Part model, mm, in its own coordinate system. A direction names the side the tool comes from. Coordinates: 2 decimals unless noted, no trailing zeros. Loops run counter-clockwise (first coordinate to the right, second up) from the corner with the lowest first, then second, coordinate; pieces in that order, holes last. Notation, with made-up numbers: M 78,81 L 110,81 A28 ccw 110,108 Z; hole C 28,29 d2. An arc over 180 degrees is marked long. Answer as a JSON object with one key per item and string values. Group by question number.
1. 3-axis set-ups, long thin cutter, end or side, ignore diameter. For faces 1 (the face through (-22.024, -6.007, -19.076)), 2 (the face through (-23, 5, 0)), 3 (the face through (39.634, 5.362, -12.932)), 4 (the face through (60.171, 0, 0)), 5 (the face through (14.57, 19.961, -10.382)): which of +Z, -Z, +X, -X, +Y, -Y reach the whole face in a straight line?
2. Drop flat-ended pins along their axis: pin 1 Ø8 at (x, y) = (33, -13.5) entering from -Z; pin 2 Ø8 at (x, z) = (-34, -16) entering from -Y; pin 3 Ø8 at (x, y) = (6, 15.5) entering from +Z. Give the stop position or say it passes through.
3. Saw through at C-C on x = -36.5. Write the cut outline in (y, z), then the cut area to 3 significant figures.
4. Saw through at B-B on z = 0. Write the cut outline in (x, y).
5. Drill centre lines: L1, parallel to X at y = 2.5, z = -3; L2, parallel to X at y = 3.5, z = 15; L3, parallel to Y at x = -2.5, z = -10. Where is each one in solid material? Low to high.
6. Saw through at D-D on z = 7.5. Write the cut outline in (x, y).
7. Saw through at A-A on y = 0. Write the cut outline in (x, z), then the cut area to 3 significant figures.
from build123d import *

# Parameters (mm, degrees)
CUT_EXTRUDE1_DEPTH      = 69.066884873
CUT_EXTRUDE1_DEPTH_BACK = 69.066884873
SKETCH2_W               = 43
SKETCH2_H               = 10


with BuildPart() as part:
    # Sketch1 → Revolve1 (revolve)
    with BuildSketch(Plane(origin=(0, 0, 0), x_dir=(1, 0, 0), z_dir=(0, 1, 0))):
        Polygon((-55.485714286, 0), (-55.485714286, 20), (10.514285714, 20), (10.514285714, 22.5), (18.514285714, 22.5), (18.514285714, 14), (60.171428571, 14), (60.171428571, 0), align=None)
    revolve(axis=Axis((60.171428571, 0, 0), (-1, 0, 0)))

    # Sketch2 → Cut-Extrude1 (cut, two sides: drawn at the far end of the back side and taken through both)
    with BuildSketch(Plane.XY.offset(-CUT_EXTRUDE1_DEPTH_BACK)):
        with Locations((-22.985714286, 0)):
            Rectangle(SKETCH2_W, SKETCH2_H)
    extrude(amount=CUT_EXTRUDE1_DEPTH + CUT_EXTRUDE1_DEPTH_BACK, mode=Mode.SUBTRACT)


solid = part.part
Outcome:
{
 "1": {"face 1": "-X", "face 2": "+Z, -Z", "face 3": "+X", "face 4": "+Z, -Z, +X, +Y, -Y", "face 5": "+X, -X"},
 "2": {"pin 1": "stops at z = -10.28", "pin 2": "stops at y = -16", "pin 3": "stops at z = 16.36"},
 "3": {"outline": "M -5,-19.36 L -5,19.36 A20 ccw Z; M 5,-19.36 A20 ccw 5,19.36 Z", "area": "861 mm²"},
 "4": {"outline": "M -55.49,-20 L 10.51,-20 L 10.51,-22.5 L 18.51,-22.5 L 18.51,-14 L 60.17,-14 L 60.17,14 L 18.51,14 L 18.51,22.5 L 10.51,22.5 L 10.51,20 L -55.49,20 Z; hole M -44.49,-5 L -1.49,-5 L -1.49,5 L -44.49,5 Z"},
 "5": {"L1": "x = -55.49 to -44.49, -1.49 to 60.17", "L2": "x = -55.49 to -44.49, -1.49 to 18.51", "L3": "y = -17.32 to -5, 5 to 17.32"},
 "6": {"outline": "M -55.49,-18.54 L 10.51,-18.54 L 10.51,-21.21 L 18.51,-21.21 L 18.51,-11.82 L 60.17,-11.82 L 60.17,11.82 L 18.51,11.82 L 18.51,21.21 L 10.51,21.21 L 10.51,18.54 L -55.49,18.54 Z; hole M -44.49,-5 L -1.49,-5 L -1.49,5 L -44.49,5 Z"},
 "7": {"outline": "M -55.49,-20 L -44.49,-20 L -44.49,20 L -55.49,20 Z; M -1.49,-20 L 10.51,-20 L 10.51,-22.5 L 18.51,-22.5 L 18.51,-14 L 60.17,-14 L 60.17,14 L 18.51,14 L 18.51,22.5 L 10.51,22.5 L 10.51,20 L -1.49,20 Z", "area": "2,450 mm²"}
}
